Source: CAD feature listing. Evaluate the final solid. Frame: model axes, mm. A direction names the side the tool comes from. Give positions to 0.01 mm unless a question says otherwise; leave off trailing zeros. Loops run counter-clockwise (first coordinate to the right, second up) from the corner with the lowest first, then second, coordinate; pieces in that order, holes last. Notation, with made-up numbers: (-12.75, -3) - (41.25, -3) arc R15 cw to (41.25, 5) - close; hole circle Ø3 at (10, 83.25). An arc over 180 degrees is marked (long way). Put each result on its own line as item: value.
```python
from build123d import *

# Parameters (mm, degrees)
BASE_FLANGE1_DEPTH  = 30
SKETCH6_W           = 15
SKETCH6_H           = 5
TAB1_DEPTH          = 0.7366
SKETCH9_R           = 3
SKETCH9_W           = 2
SKETCH9_H           = 1.993597438
BOSS_EXTRUDE1_DEPTH = 10


# Sheet-metal steps are written as plain solids
with BuildPart() as part:
    # Sketch1 → Base-Flange1 (new body)
    with BuildSketch(Plane(origin=(0, 0, 0), x_dir=(1, 0, 0), z_dir=(0, 1, 0))):
        with BuildLine():
            Line((8, 0), (1.4732, 0))
            ThreePointArc((1.4732, 0), (0.43149029, 0.43149029), (0, 1.4732))
            Line((0, 1.4732), (0, 18.5268))
            ThreePointArc((0, 18.5268), (0.43149029, 19.56850971), (1.4732, 20))
            Line((1.4732, 20), (5, 20))
            Line((5, 20), (5, 19.2634))
            Line((5, 19.2634), (1.4732, 19.2634))
            ThreePointArc((1.4732, 19.2634), (0.952345145, 19.047654855), (0.7366, 18.5268))
            Line((0.7366, 18.5268), (0.7366, 1.4732))
            ThreePointArc((0.7366, 1.4732), (0.952345145, 0.952345145), (1.4732, 0.7366))
            Line((1.4732, 0.7366), (8, 0.7366))
            Line((8, 0.7366), (8, 0))
        make_face()
    extrude(amount=BASE_FLANGE1_DEPTH)

    # Sketch6 → Tab1 (add)
    with BuildSketch(Plane(origin=(0, 0, -20), x_dir=(-1, 0, 0), z_dir=(0, 0, -1))):
        with Locations((-12.5, 27.5)):
            Rectangle(SKETCH6_W, SKETCH6_H)
    extrude(amount=-TAB1_DEPTH)

    # Sketch9 → Boss-Extrude1 (add)
    with BuildSketch(Plane.XZ.offset(-25)):
        with Locations((20, -20)):
            Circle(SKETCH9_R)
        with Locations((20, -23)):
            Rectangle(SKETCH9_W, SKETCH9_H)
    extrude(amount=BOSS_EXTRUDE1_DEPTH)


solid = part.part
```
1) Access query for faces 4 (the flat face through (20, 15, -20)), 5 (the flat face through (4.7, 21.9, -20)), 6 (the flat face through (19, 20, -23)). Directions: +Z, -Z, +X, -X, +Y, -Y. A direction counts if a zero-diameter tool reaches every point of the face in a straight line with its end or side. Return the directions, or none.
Check result:
face 4: +Z, -Z, +X, -Y
face 5: -Z, -X, +Y
face 6: -Z, -X, +Y, -Y
2) Pin query (flat end, axial travel): P1, Ø5, axis at x = 3.5, z = -9, coming from the +Y side; P2, Ø0.6, axis at y = 17, z = -19.5, coming from the +X side; P3, Ø8.5, axis at y = 8, z = -13.5, coming from the +X side; P4, Ø3, axis at x = 8, y = 16, coming from the -Z side. Return the tip coordinate at first contact, or that it passes through.
Check result:
P1: through
P2: x = 22.99
P3: x = 0.74
P4: z = -0.74
3) Section query B-B, the plane y = 12. Output: boundary loops of the cut face in (x, z), plus the area to 3 significant figures.
Check result:
outline: (0, -18.53) arc R1.47 ccw to (1.47, -20) - (5, -20) - (5, -19.26) - (1.47, -19.26) arc R0.74 cw to (0.74, -18.53) - (0.74, -1.47) arc R0.74 cw to (1.47, -0.74) - (8, -0.74) - (8, 0) - (1.47, 0) arc R1.47 ccw to (0, -1.47) - close
area: 22.5 mm²
4) Mould query, pull axis X, two halves, no side actions, for faces 1 (the flat face through (4.7, 21.9, -19.263)), 2 (the cylindrical face through (0.42, 14.79, -19.557)), 3 (the flat face through (20, 20, -23.997)). Classes: pulls with the +X half, pulls with the -X half, needs draft (parallel to the pull), parting line crosses it, or undercut.
Check result:
face 1: undercut
face 2: pulls with the -X half
face 3: needs draft
5) Section query C-C, the plane z = -13.25. Output: boundary loops of the cut face in (x, y), plus the area to 3 significant figures.
Check result:
outline: (0, 0) - (0.74, 0) - (0.74, 30) - (0, 30) - close
area: 22.1 mm²
6) Material intervals for line 1 along Z through (x, y) = (3.25, 22); line 2 along X through (y, z) = (28.5, -12.5); line 3 along Z through (x, y) = (7.25, 15.25), sorted ascending. Write a range as [from, to].
Check result:
line 1: [-20, -19.26], [-0.74, 0]
line 2: [0, 0.74]
line 3: [-0.74, 0]
7) Section query A-A, the plane x = 3. Output: boundary loops of the cut face in (y, z).
Check result:
outline: (0, -20) - (30, -20) - (30, -19.26) - (0, -19.26) - close; (0, -0.74) - (30, -0.74) - (30, 0) - (0, 0) - close
